from build123d import *

# Parameters (mm, degrees)
BOSS_EXTRUDE1_DEPTH  = 2.54
BOSS_EXTRUDE2_DEPTH  = 30.48
CUT_EXTRUDE2_DEPTH   = 95.827847835
BOSS_EXTRUDE4_DEPTH  = 3.81
BOSS_EXTRUDE5_START  = 2
BOSS_EXTRUDE5_DEPTH  = 2.54
CHAMFER4_SIZE        = 0.762
BOSS_EXTRUDE6_DEPTH  = 3.81
M3_CLEARANCE_HOLE1_D = 3.4
SKETCH13_R           = 4.445
CUT_EXTRUDE3_DEPTH   = 2.032
BOSS_EXTRUDE3_DEPTH  = 3.81
CHAMFER2_SIZE        = 3.81
BOSS_EXTRUDE10_DEPTH = 33.02


with BuildPart() as part:
    # Sketch1 → Boss-Extrude1 (new body)
    with BuildSketch(Plane(origin=(0, 0, 0), x_dir=(1, 0, 0), z_dir=(0, 1, 0))):
        Polygon((-36.195, 66.167), (36.195, 66.167), (60.706, 41.656), (60.706, -41.656), (36.195, -66.167), (-36.195, -66.167), (-60.706, -41.656), (-60.706, 41.656), align=None)
    extrude(amount=BOSS_EXTRUDE1_DEPTH)

    # Sketch5 → Boss-Extrude2 (add)
    with BuildSketch(Plane(origin=(0, 2.54, 0), x_dir=(1, 0, 0), z_dir=(0, 1, 0))):
        Polygon((60.706, -41.656), (60.706, 41.656), (36.195, 66.167), (-36.195, 66.167), (-60.706, 41.656), (-60.706, -41.656), (-58.166, -41.656), (-58.166, 40.603897552), (-35.142897552, 63.627), (35.142897552, 63.627), (58.166, 40.603897552), (58.166, -41.656), align=None)
    extrude(amount=BOSS_EXTRUDE2_DEPTH)

    # Sketch8 → Cut-Extrude2 (cut, through all)
    with BuildSketch(Plane(origin=(0, 2.54, 0), x_dir=(1, 0, 0), z_dir=(0, 1, 0))):
        Polygon((-58.166, -44.196), (-36.195, -66.167), (-17.145, -66.167), (-39.116, -44.196), align=None)
    extrude(amount=-CUT_EXTRUDE2_DEPTH, mode=Mode.SUBTRACT)

    # Sketch9 → Boss-Extrude4 (add)
    with BuildSketch(Plane(origin=(0, 6.35, 0), x_dir=(1, 0, 0), z_dir=(0, 1, 0))):
        Polygon((-58.166, 40.603897552), (-35.142897552, 63.627), (-31.550795103, 63.627), (-58.166, 37.011795103), align=None)
        Polygon((31.550795103, 63.627), (58.166, 37.011795103), (58.166, 40.603897552), (35.142897552, 63.627), align=None)
    extrude(amount=-BOSS_EXTRUDE4_DEPTH)

    # Sketch9<3> → Boss-Extrude5 (add)
    with BuildSketch(Plane(origin=(0, 6.35, 0), x_dir=(1, 0, 0), z_dir=(0, 1, 0)).offset(BOSS_EXTRUDE5_START)):
        Polygon((-58.166, 40.603897552), (-35.142897552, 63.627), (-31.550795103, 63.627), (-58.166, 37.011795103), align=None)
        Polygon((31.550795103, 63.627), (58.166, 37.011795103), (58.166, 40.603897552), (35.142897552, 63.627), align=None)
    extrude(amount=BOSS_EXTRUDE5_DEPTH)

    # Chamfer4
    chamfer4_edges = [part.edges().sort_by_distance(p)[0] for p in [
        (-44.858397552, 10.89, -50.319397552),
        (-44.858397552, 8.35, -50.319397552),
        (44.858397552, 10.89, -50.319397552),
        (44.858397552, 8.35, -50.319397552),
        (-44.858397552, 6.35, -50.319397552),
        (44.858397552, 6.35, -50.319397552),
    ]]
    chamfer(chamfer4_edges, length=CHAMFER4_SIZE)

    # Sketch10 → Boss-Extrude6 (add)
    with BuildSketch(Plane(origin=(0, 2.54, 0), x_dir=(1, 0, 0), z_dir=(0, 1, 0))):
        Polygon((42.582385309, -56.187512242), (35.142897552, -63.627), (24.621873067, -63.627), (24.621873067, -56.187512242), (29.882385309, -50.927), (37.321873067, -50.927), align=None)
    extrude(amount=BOSS_EXTRUDE6_DEPTH)

    # M3 Clearance Hole1 (through all)
    with Locations(Plane(origin=(0, 6.35, 0), x_dir=(1, 0, 0), z_dir=(0, 1, 0))):
        with Locations((32.258, -57.277)):
            Hole(M3_CLEARANCE_HOLE1_D / 2)

    # Sketch13 → Cut-Extrude3 (cut)
    with BuildSketch(Plane.XZ):
        with Locations(Location((32.258, 57.277, 0), (0, 0, 270))):
            Circle(SKETCH13_R)
    extrude(amount=-CUT_EXTRUDE3_DEPTH, mode=Mode.SUBTRACT)

    # Sketch7 → Boss-Extrude3 (add)
    with BuildSketch(Plane(origin=(0, 33.02, 0), x_dir=(1, 0, 0), z_dir=(0, 1, 0))):
        Polygon((-58.166, -41.656), (-54.356, -41.656), (-54.356, 39.025743879), (-33.564743879, 59.817), (33.564743879, 59.817), (54.356, 39.025743879), (54.356, -41.656), (58.166, -41.656), (58.166, 40.603897552), (35.142897552, 63.627), (-35.142897552, 63.627), (-58.166, 40.603897552), align=None)
    extrude(amount=-BOSS_EXTRUDE3_DEPTH)

    # Chamfer2
    chamfer2_edges = [part.edges().sort_by_distance(p)[0] for p in [
        (54.356, 29.21, 1.315128061),
        (43.960371939, 29.21, -49.421371939),
        (0, 29.21, -59.817),
        (-43.960371939, 29.21, -49.421371939),
        (-54.356, 29.21, 1.315128061),
    ]]
    chamfer(chamfer2_edges, length=CHAMFER2_SIZE - 0.0001)  # a hair under: the kernel refuses the full size

    # Sketch14 → Boss-Extrude10 (add)
    with BuildSketch(Plane.XZ):
        Polygon((-8.255, -66.167), (-8.255, -71.247), (-10.795, -71.247), (-15.875, -66.167), align=None)
        Polygon((10.795, -71.247), (15.875, -66.167), (8.255, -66.167), (8.255, -71.247), align=None)
    extrude(amount=-BOSS_EXTRUDE10_DEPTH)


solid = part.part
Verification items for the finished model (mm, model axes). A direction names the side the tool comes from. Give positions to 0.01 mm unless a question says otherwise; leave off trailing zeros. Write each loop counter-clockwise with the first axis right and the second up, starting at its lowest first coordinate (ties: lowest second). Pieces come first, ordered by that corner, then holes. Notation, with made-up numbers: (72, 15.25) - (107, 15.25) arc R28 ccw to (107, 47.25) - close; hole circle Ø8 at (4.5, 66). An arc over 180 degrees is marked (long way). Answer as CSV lines item,"result". Start each with the question number.
1. Sectioned sample at A-A (y = 27.5). Record the boundary of the cut face in (x, z) (3 decimals), then the cut area to 3 significant figures.
2. Draft check along X on faces 1 (the face through (13.3, 16.28, -68.74)), 2 (the face through (-44.945, 5.974, -50.779)), 3 (the face through (34, 4, 50.927)), 4 (the face through (46, 10.89, -52)). Enter one of: pulls with the +X half, pulls with the -X half, needs draft (parallel to the pull), parting line crosses it, or undercut.
3. Depth check by flat-ended pin: pin 1 (6 mm diameter, centred on x = 25.5, y = 15, fed in from -Z); pin 2 (1.3 mm diameter, centred on x = -48.5, y = 1, fed in from +Z); pin 3 (5 mm diameter, centred on x = 57.5, y = 11.5, fed in from +Z). Enter the tip coordinate at first touch or a pass-through.
4. Set-up check for faces 5 (the face through (-59, 18, 41.656)), 6 (the face through (32, 2.032, 55)), 7 (the face through (0, 16, -66.167)), 8 (the face through (44.945, 5.974, -50.779)): record each of +Z, -Z, +X, -X, +Y, -Y from which the full face is reachable in a straight line by a thin tool's end or side.
5. Thickness scan on line 1 (X direction, y = 18, z = -13.5); line 2 (Y direction, x = 36, z = 50.5); line 3 (Z direction, x = -10, y = 27.5). Record the ranges inside material, lowest first.
Derived:
1,outline,"(-60.706, -41.656) - (-36.195, -66.167) - (-15.875, -66.167) - (-10.795, -71.247) - (-8.255, -71.247) - (-8.255, -66.167) - (8.255, -66.167) - (8.255, -71.247) - (10.795, -71.247) - (15.875, -66.167) - (36.195, -66.167) - (60.706, -41.656) - (60.706, 41.656) - (58.166, 41.656) - (58.166, -40.604) - (35.143, -63.627) - (-35.143, -63.627) - (-58.166, -40.604) - (-58.166, 41.656) - (-60.706, 41.656) - close"
1,area,"824 mm²"
2,face 1,"pulls with the +X half"
2,face 2,"undercut"
2,face 3,"needs draft"
2,face 4,"undercut"
3,pin 1,"z = -66.17"
3,pin 2,"z = 44.2"
3,pin 3,"z = 41.66"
4,face 5,"+Z, +X, -X, +Y"
4,face 6,"-Y"
4,face 7,"-Z, +Y, -Y"
4,face 8,"none"
5,line 1,"-60.71 to -58.17, 58.17 to 60.71"
5,line 2,"0 to 2.54"
5,line 3,"-71.25 to -63.63"
